from build123d import *

# Parameters (mm, degrees)
SKETCH1_W           = 31.6
SKETCH1_H           = 15.8
BOSS_EXTRUDE1_DEPTH = 9.4
SKETCH2_W           = 31.6
SKETCH2_H           = 13
CUT_EXTRUDE1_DEPTH  = 1.7
BOSS_EXTRUDE2_DEPTH = 20
BOSS_EXTRUDE3_DEPTH = 20
SKETCH5_R           = 2.35
BOSS_EXTRUDE4_DEPTH = 1.5


with BuildPart() as part:
    # Sketch1 → Boss-Extrude1 (new body)
    with BuildSketch(Plane(origin=(0, 0, 0), x_dir=(1, 0, 0), z_dir=(0, 1, 0))):
        with Locations((-1.354285714, -0.451428571)):
            Rectangle(SKETCH1_W, SKETCH1_H)
    extrude(amount=BOSS_EXTRUDE1_DEPTH)

    # Sketch2 → Cut-Extrude1 (cut)
    with BuildSketch(Plane(origin=(0, 0, 0), x_dir=(-1, 0, 0), z_dir=(0, -1, 0))):
        with Locations((1.354285714, -0.451428571)):
            Rectangle(SKETCH2_W, SKETCH2_H)
    extrude(amount=-CUT_EXTRUDE1_DEPTH, mode=Mode.SUBTRACT)

    # Sketch3 → Boss-Extrude2 (add)
    with BuildSketch(Plane(origin=(0, 0, -7.448571429), x_dir=(-1, 0, 0), z_dir=(0, 0, -1))):
        Polygon((-3.645714286, 9.4), (1.354285714, 3.2), (6.354285714, 9.4), align=None)
    extrude(amount=BOSS_EXTRUDE2_DEPTH)

    # Sketch4 → Boss-Extrude3 (add)
    with BuildSketch(Plane.XY.offset(8.351428571)):
        Polygon((-6.354285714, 9.4), (-1.354285714, 3.2), (3.645714286, 9.4), align=None)
    extrude(amount=BOSS_EXTRUDE3_DEPTH)

    # Sketch5 → Boss-Extrude4 (add)
    with BuildSketch(Plane(origin=(0, 9.4, 0), x_dir=(1, 0, 0), z_dir=(0, 1, 0))):
        with Locations(Location((10.645714286, -4.451428571, 0), (0, 0, 270))):
            Circle(SKETCH5_R)
        with Locations(Location((2.645714286, -4.451428571, 0), (0, 0, 270))):
            Circle(SKETCH5_R)
        with Locations(Location((-5.354285714, -4.451428571, 0), (0, 0, 270))):
            Circle(SKETCH5_R)
        with Locations(Location((-13.354285714, -4.451428571, 0), (0, 0, 270))):
            Circle(SKETCH5_R)
        with Locations(Location((2.645714286, 3.548571429, 0), (0, 0, 270))):
            Circle(SKETCH5_R)
        with Locations(Location((-5.354285714, 3.548571429, 0), (0, 0, 270))):
            Circle(SKETCH5_R)
        with Locations(Location((-13.354285714, 3.548571429, 0), (0, 0, 270))):
            Circle(SKETCH5_R)
        with Locations(Location((10.645714286, 3.548571429, 0), (0, 0, 270))):
            Circle(SKETCH5_R)
    extrude(amount=BOSS_EXTRUDE4_DEPTH)


solid = part.part
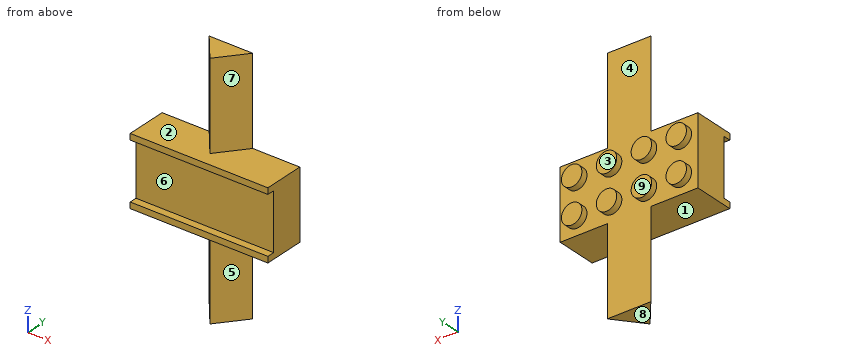
Design review of the part built by this model. Coordinates are the model's own, in mm. Face numbers are marked on the shaded views. A direction names the side the tool comes from. Round coordinates to 2 decimals unless told otherwise and drop trailing zeros. Write each loop counter-clockwise with the first axis right and the second up, starting at its lowest first coordinate (ties: lowest second). Pieces come first, ordered by that corner, then holes. Notation, with made-up numbers: (20.25, 67) - (43.25, 67) arc R21 cw to (43.25, 77) - close; hole circle Ø1 at (-15.5, 9). An arc over 180 degrees is marked (long way). Use a Markdown table: item, result. Add a question column.
1. For the marked faces 5, 6, 7, 8 and 9, list the 3-axis set-ups (+Z, -Z, +X, -X, +Y, -Y) from which the entire face can be reached by the end or side of a thin tool; tool diameter is ignored.
2. We need section D-D (y = 7.5). State the section outline as (x, z) points, then the cut area to 3 significant figures.
3. We need section B-B (x = 6.5). State the section outline as (y, z) points.
4. Mouldability with a two-part tool opening along Z and no side actions: class the marked faces 1, 2, 3 and 4 as +Z half, -Z half, draft (parallel to the pull), parting line (faces both ways), or undercut.
5. Wall thickness on probe 1 along X at (y, z) = (9.5, 5); probe 2 along Z at (x, y) = (-13.5, 1); probe 3 along Z at (x, y) = (12, 9): over which ranges is each line inside the solid? List them lowest first.
6. We need section C-C (z = 4). State the section outline as (x, y) points.
7. Clearance check with flat-ended pins moving along their axes: pin 1 (5 mm diameter, centred on x = -10, y = 1.5, fed in from -Z); pin 2 (5 mm diameter, centred on x = -11, z = -19, fed in from +Y); pin 3 (4 mm diameter, centred on x = 4.5, z = 2.5, fed in from -Y); pin 4 (1.9 mm diameter, centred on x = -9, y = 1, fed in from +Z). State where each tip first meets the part, or that it passes through.
8. We need section A-A (y = 10.25). State the section outline as (x, z) points.
Output:
| question | item | result |
|---|---|---|
| 1 | face 5 | -Z, +X, -Y |
| 1 | face 6 | +X, -X, -Y |
| 1 | face 7 | +Z, +X, -Y |
| 1 | face 8 | -Z, +X, -X, +Y, -Y |
| 1 | face 9 | +Z, -Z, +X, -X, +Y |
| 2 | outline | (-17.15, -7.45) - (-4.82, -7.45) - (-4.82, -27.45) - (2.11, -27.45) - (2.11, -7.45) - (14.45, -7.45) - (14.45, 8.35) - (2.11, 8.35) - (2.11, 28.35) - (-4.82, 28.35) - (-4.82, 8.35) - (-17.15, 8.35) - close |
| 2 | area | 777 mm2 |
| 3 | outline | (0, -7.45) - (9.4, -7.45) - (9.4, 8.35) - (0, 8.35) - (0, 6.95) - (1.7, 6.95) - (1.7, -6.05) - (0, -6.05) - close |
| 4 | face 1 | -Z half |
| 4 | face 2 | +Z half |
| 4 | face 3 | draft |
| 4 | face 4 | undercut |
| 5 | probe 1 | x = -15.64 to -11.07, -7.64 to -3.07, 0.36 to 4.93, 8.36 to 12.93 |
| 5 | probe 2 | z = -7.45 to -6.05, 6.95 to 8.35 |
| 5 | probe 3 | z = -7.45 to 8.35 |
| 6 | outline | (-17.15, 1.7) - (14.45, 1.7) - (14.45, 9.4) - (12.95, 9.4) - (12.95, 10.9) - (8.34, 10.9) - (8.34, 9.4) - (4.95, 9.4) - (4.95, 10.9) - (0.34, 10.9) - (0.34, 9.4) - (-3.05, 9.4) - (-3.05, 10.9) - (-7.66, 10.9) - (-7.66, 9.4) - (-11.05, 9.4) - (-11.05, 10.9) - (-15.66, 10.9) - (-15.66, 9.4) - (-17.15, 9.4) - close |
| 7 | pin 1 | stops at z = -7.45 |
| 7 | pin 2 | passes through |
| 7 | pin 3 | stops at y = 1.7 |
| 7 | pin 4 | stops at z = 8.35 |
| 8 | outline | circle Ø4.7 at (-13.35, -3.55); circle Ø4.7 at (-13.35, 4.45); circle Ø4.7 at (-5.35, -3.55); circle Ø4.7 at (-5.35, 4.45); circle Ø4.7 at (2.65, -3.55); circle Ø4.7 at (2.65, 4.45); circle Ø4.7 at (10.65, -3.55); circle Ø4.7 at (10.65, 4.45) |
